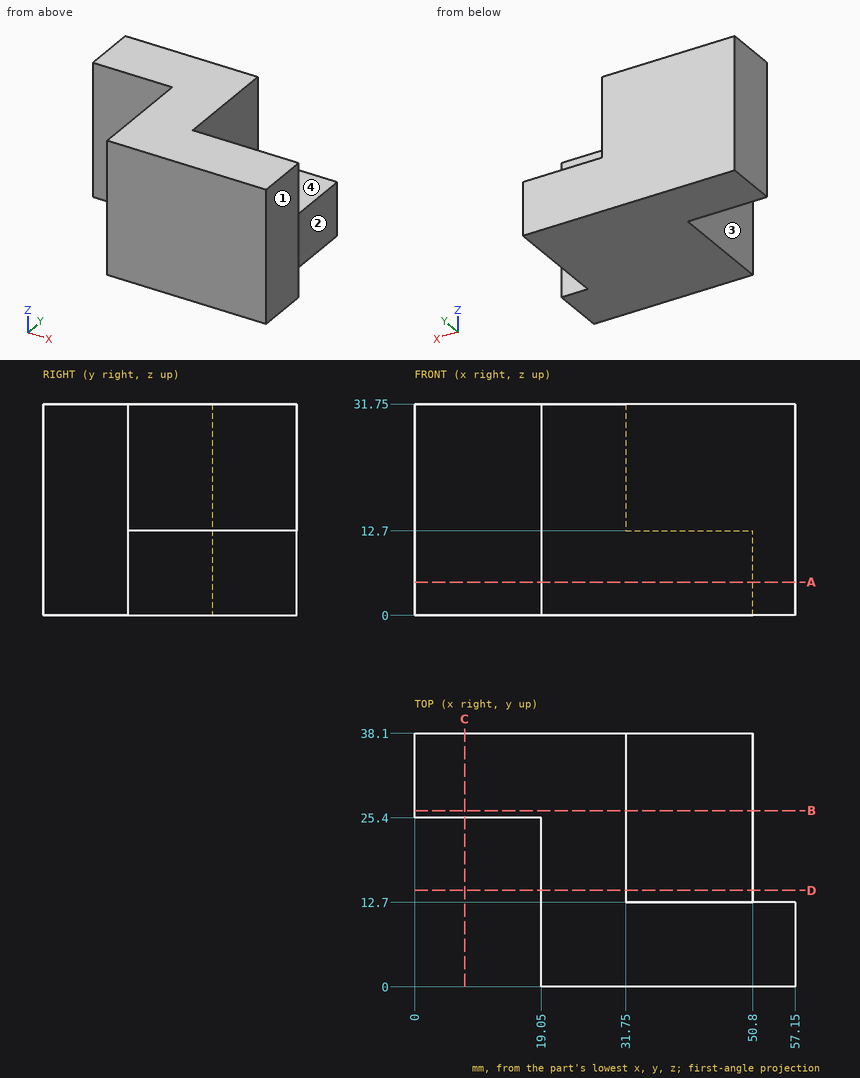
Design review of the part shown in the three views and the two pictorial views. Dimensions are in mm from the part's minimum x, y and z. A direction names the side the tool comes from. Round coordinates to 2 decimals unless told otherwise and drop trailing zeros. Loops run counter-clockwise (first coordinate to the right, second up) from the corner with the lowest first, then second, coordinate; pieces in that order, holes last. Notation, with made-up numbers: M -1.75,-33 L 52.25,-33 A19 ccw 52.25,3 Z; hole C 35,69.5 d1. An arc over 180 degrees is marked long. Answer as a JSON object with one key per item and string values.
Item 1: We need section C-C on x = 7.5. Give the boundary of the cut face in (y, z), and give its area (3 significant figures).
Answer sheet:
{"outline": "M 25.4,0 L 38.1,0 L 38.1,31.75 L 25.4,31.75 Z", "area": "403 mm^2"}
Item 2: We need section A-A on z = 5. Give the boundary of the cut face in (x, y).
Answer sheet:
{"outline": "M 0,25.4 L 19.05,25.4 L 19.05,0 L 57.15,0 L 57.15,12.7 L 50.8,12.7 L 50.8,38.1 L 0,38.1 Z"}
Item 3: We need section B-B on y = 26.5. Give the boundary of the cut face in (x, z), and give its area (3 significant figures).
Answer sheet:
{"outline": "M 0,0 L 50.8,0 L 50.8,12.7 L 31.75,12.7 L 31.75,31.75 L 0,31.75 Z", "area": "1,250 mm^2"}
Item 4: We need section D-D on y = 14.5. Give the boundary of the cut face in (x, z), and give its area (3 significant figures).
Answer sheet:
{"outline": "M 19.05,0 L 50.8,0 L 50.8,12.7 L 31.75,12.7 L 31.75,31.75 L 19.05,31.75 Z", "area": "645 mm^2"}
Item 5: Clearance check with flat-ended pins moving along their axes: P1, Ø3, axis at y = 23.5, z = 22, coming from the +X side; P2, Ø5, axis at x = 10.5, z = 12, coming from the -Y side; P3, Ø5, axis at y = 12.5, z = 18, coming from the -X side. State where each tip first meets the part, or that it passes through.
Answer sheet:
{"P1": "stops at x = 31.75", "P2": "stops at y = 25.4", "P3": "stops at x = 19.05"}
Item 6: Wall thickness on L1, parallel to Y at x = 8, z = 5; L2, parallel to X at y = 26, z = 19; L3, parallel to Y at x = 32.5, z = 27.5: over which ranges is each line inside the solid? List them lowest first. Write a range as from..to.
Answer sheet:
{"L1": "y = 25.4..38.1", "L2": "x = 0..31.75", "L3": "y = 0..12.7"}
Item 7: Machinability: for the marked faces 1, 2, 3 and 4, which of the approach directions +Z, -Z, +X, -X, +Y, -Y give a long, thin tool a straight path to every point of the face, cutting with its end or side? Answer none if there is none.
Answer sheet:
{"face 1": "+Z, -Z, +X, +Y, -Y", "face 2": "+Z, -Z, +X, +Y", "face 3": "+Z, -Z, -X, -Y", "face 4": "+Z, +X, +Y"}
